Autodesk Inventor part; units mm, degrees
ref_plane "YZ Plane" through (0, 0, 0) normal (1, 0, 0) x (0, 1, 0)
ref_plane "XZ Plane" through (0, 0, 0) normal (0, 1, 0) x (-1, 0, 0)
ref_plane "XY Plane" through (0, 0, 0) normal (0, 0, 1) x (1, 0, 0)
sketch "Sketch1" plane through (0, 0, 0) normal (0, 1, 0) x (-1, 0, 0)
  line L0 (0, 0) -> (-56, 0)
  line L1 (-56, 0) -> (-56, -85.25)
  line L2 (-56, -85.25) -> (0, -85.25)
  line L3 (0, -85.25) -> (0, 0)
  dimension "d0" = 56
  dimension "d1" = 85.25
extrude "Extrusion1" add sketch "Sketch1" along normal blind 2
sketch "Sketch2" plane through (0, 2, 0) normal (0, 1, 0) x (1, 0, 0)
  line L0 (0, 85.25) -> (0, 0)
  line L1 (0, 0) -> (56, 0)
  line L2 (56, 0) -> (56, 85.25)
  line L3 (56, 85.25) -> (0, 85.25)
  line L4 (0, 85.25) -> (0, 0)
  line L5 (0, 0) -> (56, 0)
  line L6 (56, 0) -> (56, 85.25)
  line L7 (56, 85.25) -> (0, 85.25)
  line L8 (0, 85.25) -> (0, 0)
  line L9 (57, -1) -> (-1, -1)
  line L10 (-1, -1) -> (-1, 86.25)
  line L11 (-1, 86.25) -> (57, 86.25)
  line L12 (57, 86.25) -> (57, -1)
  dimension "d5" = 1
extrude "Extrusion2" add sketch "Sketch2" along normal blind 3.5 and the other way blind 2
fillet "Fillet1" radius 3 8 edges at (-1, 2.75, 1) (57, 2.75, 1) (57, 2.75, -86.25) (-1, 2.75, -86.25) (56, 3.75, 0) (0, 3.75, 0) (56, 3.75, -85.25) (0, 3.75, -85.25)
sketch "Sketch3" plane through (0, 2, 0) normal (0, 1, 0) x (1, 0, 0)
  line L0 (2, -1) -> (54, -1)
  line L1 (53, 0) -> (3, 0)
  line L2 (0, 3) -> (0, 82.25)
  line L3 (-1, 83.25) -> (-1, 2)
  line L4 (-1, 2) -> (-1, 83.25)
  arc A0 (0, 3) -> (3, 0) centre (3, 3) ccw
  line L5 (0, 82.25) -> (0, 3)
  line L6 (0, 3) -> (0, 0)
  line L7 (0, 0) -> (3, 0)
  line L8 (3, 0) -> (3.5, 0)
  line L9 (3.5, 0) -> (3.5, 3.5)
  circle A1 centre (3.5, 3.5) radius 1.25
  arc A2 (53, 0) -> (56, 3) centre (53, 3) ccw
  line L10 (56, 3) -> (56, 0)
  line L11 (56, 0) -> (53, 0)
  line L12 (53, 0) -> (52.5, 0)
  line L13 (52.5, 0) -> (52.5, 3.5)
  circle A3 centre (52.5, 3.5) radius 1.25
  arc A4 (3, 85.25) -> (0, 82.25) centre (3, 82.25) ccw
  line L14 (0, 82.25) -> (0, 85.25)
  line L15 (0, 85.25) -> (3, 85.25)
  line L16 (3, 85.25) -> (53, 85.25)
  circle A5 centre (3.5, 61.5) radius 1.25
  line L17 (56, 82.25) -> (56, 3)
  line L18 (56, 82.25) -> (56, 85.25)
  line L19 (56, 85.25) -> (56.5, 85.25)
  arc A6 (56, 82.25) -> (53, 85.25) centre (53, 82.25) ccw
  circle A7 centre (52.5, 61.5) radius 1.25
  dimension "d9" = 0.5
  dimension "d10" = 3.5
  dimension "d11" = 2.5
  dimension "d12" = 0.5
  dimension "d13" = 3.5
  dimension "d14" = 2.5
  dimension "d17" = 2.5
  dimension "d21" = 2.5
  dimension "d24" = 61.5
  dimension "d25" = 3.5
  dimension "d26" = 61.5
  dimension "d27" = 3.5
extrude "Extrusion3" cut sketch "Sketch3" against normal up to next contours A1 | A3 | A5 | A7
sketch "Sketch4" plane through (0, 2, 0) normal (0, 1, 0) x (1, 0, 0)
  circle A0 centre (3.5, 3.5) radius 1.25
  arc A1 (0, 3) -> (3, 0) centre (3, 3) ccw
  arc A2 (7, 3.5) -> (3.5, 7) centre (3.5, 3.5) ccw
  line L0 (3, 0) -> (53, 0)
  line L1 (3.5, 7) -> (0, 7)
  line L2 (0, 82.25) -> (0, 3)
  line L3 (7, 3.5) -> (7, 0)
  circle A3 centre (3.5, 3.5) radius 1.25
  circle A4 centre (52.5, 3.5) radius 1.25
  line L4 (56, 82.25) -> (56, 3)
  line L5 (53, 0) -> (3, 0)
  circle A5 centre (56.5, 3.5) radius 1.25
  circle A6 centre (3.5, 61.5) radius 1.25
  circle A7 centre (52.5, 61.5) radius 1.25
  arc A8 (3.5, 58) -> (3.5, 65) centre (3.5, 61.5) ccw
  arc A9 (52.5, 65) -> (52.5, 58) centre (52.5, 61.5) ccw
  line L6 (3.5, 65) -> (0, 65)
  line L7 (3.5, 58) -> (0, 58)
  line L8 (52.5, 65) -> (56, 65)
  line L9 (52.5, 58) -> (56, 58)
  circle A10 centre (3.5, 61.5) radius 1.25
  circle A11 centre (52.5, 61.5) radius 1.25
  circle A12 centre (3.5, 61.5) radius 1.25
  circle A13 centre (3.5, 3.5) radius 1.25
  circle A14 centre (52.5, 3.5) radius 1.25
  circle A15 centre (52.5, 61.5) radius 1.25
  arc A16 (3, 85.25) -> (0, 82.25) centre (3, 82.25) ccw
  line L10 (0, 82.25) -> (0, 3)
  arc A17 (0, 3) -> (3, 0) centre (3, 3) ccw
  line L11 (3, 0) -> (53, 0)
  arc A18 (53, 0) -> (56, 3) centre (53, 3) ccw
  line L12 (56, 3) -> (56, 82.25)
  arc A19 (56, 82.25) -> (53, 85.25) centre (53, 82.25) ccw
  line L13 (53, 85.25) -> (3, 85.25)
  arc A20 (53, 0) -> (56, 3) centre (53, 3) ccw
  arc A21 (52.5, 7) -> (49, 3.5) centre (52.5, 3.5) ccw
  line L14 (52.5, 7) -> (56, 7)
  line L15 (49, 3.5) -> (49, 0)
  point P0 (0, 0)
  dimension "d31" = 7
  dimension "d32" = 7
  dimension "d33" = 7
extrude "Extrusion4" add sketch "Sketch4" along normal blind 2 contours L2 L1 A2 L3 L0 A1 | L2 L6 A8 L7 | L15 A21 L14 L4 A5 A18 L0 | A5 L4 A18 | L9 A9 L8 L4 picked at (55.9186, 4.05)
sketch "Sketch5" plane through (57, 0, -83.25) normal (1, 0, 0) x (0, 0, -1)
  line L0 (-81.25, 0) -> (-81.25, 5.5)
  line L1 (0, 0) -> (0, 5.5)
  line L2 (-81.25, 0) -> (0, 0)
  line L3 (0, 0) -> (0, 2)
  line L4 (0, 2) -> (-81.25, 2)
  line L5 (-81.25, 2) -> (-81.25, 0)
  point P0 (-83.25, 0)
  dimension "d36" = 2
extrude "Extrusion5" add sketch "Sketch5" along normal blind 3
sketch "Sketch6" plane through (-1, 0, -83.25) normal (-1, 0, 0) x (0, 0, 1)
  line L0 (81.25, 2) -> (0, 2)
  line L1 (81.25, 0) -> (0, 0)
  line L2 (81.25, 5.5) -> (81.25, 0)
  line L3 (0, 0) -> (0, 5.5)
  point P0 (83.25, 0)
extrude "Extrusion6" add sketch "Sketch6" along normal blind 3
sketch "Sketch7" plane through (0, 0, 0) normal (0, -1, 0) x (1, 0, 0)
  circle A0 centre (3.5, -3.5) radius 1.25
  circle A1 centre (52.5, -3.5) radius 1.25
  circle A2 centre (52.5, -61.5) radius 1.25
  circle A3 centre (3.5, -61.5) radius 1.25
  circle A4 centre (3.5, -3.5) radius 3
  circle A5 centre (52.5, -3.5) radius 3
  circle A6 centre (52.5, -61.5) radius 3
  circle A7 centre (3.5, -61.5) radius 3
  point P0 (0, 0)
  dimension "d41" = 6
  dimension "d42" = 6
  dimension "d43" = 6
  dimension "d44" = 6
extrude "Extrusion7" cut sketch "Sketch7" against normal blind 2
properties part number "pi-holder"
For this review, take the finished solid that the model builds, in its own axes (mm). A direction names the side the tool comes from. Round coordinates to 2 decimals unless told otherwise and drop trailing zeros. Order: outer loops, then holes, each group sorted by start corner. A loop starts at its lowest first (then second) coordinate and runs counter-clockwise, first axis right, second up. Notation, with made-up numbers: (68.5, -24.75) -> (87.5, -24.75) arc R10 ccw to (87.5, -10.75) -> close; hole circle Ø5 at (-15.75, 19). An arc over 180 degrees is marked (long way). Put each result on its own line as item: value.
Q1. Add section D-D on z = -47. Write out the cut boundary in (x, y).
Check result:
outline: (-4, 0) -> (60, 0) -> (60, 2) -> (57, 2) -> (57, 5.5) -> (56, 5.5) -> (56, 2) -> (0, 2) -> (0, 5.5) -> (-1, 5.5) -> (-1, 2) -> (-4, 2) -> close
Q2. For probe 1 along X at (y, z) = (3.3, -61.5); probe 2 along Z at (x, y) = (3.5, 3.1); probe 3 along X at (y, z) = (2.5, -22), list the stretches that pass through material, from the lowest coordinate up. Write a range as [from, to].
Check result:
probe 1: [-1, 2.25], [4.75, 7], [49, 51.25], [53.75, 57]
probe 2: [-86.25, -85.25], [-65, -62.75], [-60.25, -58], [-7, -4.75], [-2.25, 1]
probe 3: [-1, 0], [56, 57]
Q3. Add section A-A on z = -61.5. State how many separate pieces and enclosed holes the cut face has, plus the area to 3 significant figures.
Check result:
separate pieces: 3
enclosed holes: 0
area: 129 mm2
Q4. Mouldability with a two-part tool opening along X and no side actions: class faces 5 (the flat face through (54, 3, -58)), 6 (the cylindrical face through (-0.14, 2.71, -85.35)), 7 (the flat face through (28, 0, -42)) as pulls with the +X half, pulls with the -X half, needs draft (parallel to the pull), parting line crosses it, or undercut.
Check result:
face 5: undercut
face 6: pulls with the -X half
face 7: needs draft
Q5. Machinability: for faces 1 (the flat face through (-2, 2, -42)), 2 (the cylindrical face through (49, 3, -61.4)), 3 (the cylindrical face through (56.14, 2.79, -85.35)), 4 (the cylindrical face through (0.5, 1, -3.4)), which of the approach directions +Z, -Z, +X, -X, +Y, -Y give a long, thin tool a straight path to every point of the face, cutting with its end or side? Answer none if there is none.
Check result:
face 1: +Z, -Z, -X, +Y
face 2: +Y
face 3: -Z, +X, +Y, -Y
face 4: -Y
Q6. Insertion check: pin 1 Ø3.5 at (x, z) = (53.5, -4.5) entering from +Y; pin 2 Ø1 at (y, z) = (2.5, -1.5) entering from +X; pin 3 Ø0.6 at (x, y) = (58.5, 0.5) entering from -Z; pin 4 Ø1.5 at (x, z) = (3.5, -3.5) entering from -Y. Each pin has a flat end and moves straight along its axis. Give the tip position at first contact, or say it passes through.
Check result:
pin 1: y = 4
pin 2: x = 57
pin 3: z = -83.25
pin 4: through
Q7. Add section B-B on y = 0.95. Write out the cut boundary in (x, z), plus the area to 3 significant figures.
Check result:
outline: (-4, -83.25) -> (-1, -83.25) arc R3 ccw to (2, -86.25) -> (54, -86.25) arc R3 ccw to (57, -83.25) -> (60, -83.25) -> (60, -2) -> (57, -2) arc R3 ccw to (54, 1) -> (2, 1) arc R3 ccw to (-1, -2) -> (-4, -2) -> close; hole circle Ø6 at (3.5, -61.5); hole circle Ø6 at (3.5, -3.5); hole circle Ø6 at (52.5, -61.5); hole circle Ø6 at (52.5, -3.5)
area: 5,430 mm2
Q8. Add section C-C on x = 10. Write out the cut boundary in (y, z).
Check result:
outline: (0, -86.25) -> (5.5, -86.25) -> (5.5, -85.25) -> (2, -85.25) -> (2, 0) -> (5.5, 0) -> (5.5, 1) -> (0, 1) -> close
